Could you check a few things on this model? Use its own coordinates, in mm. A direction names the side the tool comes from. Coordinates: 2 decimals unless noted, no trailing zeros. Order: outer loops, then holes, each group sorted by start corner. A loop starts at its lowest first (then second) coordinate and runs counter-clockwise, first axis right, second up. Notation, with made-up numbers: (-33.75, 33) - (-14.75, 33) arc R23 cw to (-14.75, 56) - close; hole circle Ø6 at (-15.75, 74.5). An arc over 180 degrees is marked (long way). One line per item, written item: value.
from build123d import *

# Parameters (mm, degrees)
BODY_SKETCH_W       = 32
BODY_SKETCH_H       = 26.7
BODY_DEPTH          = 12.7
NUT_X_SKETCH_W      = 16.75
NUT_X_SKETCH_H      = 9.45
NUT_X_SKETCH_2_W    = 16.75
NUT_X_SKETCH_2_H    = 9.45
SOCKET_X_SKETCH_W   = 17.8
SOCKET_X_SKETCH_H   = 4.7625
SOCKET_X_SKETCH_2_W = 17.8
SOCKET_X_SKETCH_2_H = 4.7625


with BuildPart() as part:
    # Body Sketch → Body (new, symmetric)
    with BuildSketch(Plane.XY):
        with Locations((0, 0.65)):
            Rectangle(BODY_SKETCH_W, BODY_SKETCH_H)
    extrude(amount=BODY_DEPTH, both=True)

    # Nut _X Sketch → Nut _X (revolve)
    with BuildSketch(Plane.XY, mode=Mode.PRIVATE) as nut_x_sk:
        with Locations((24.375, 4.725)):
            Rectangle(NUT_X_SKETCH_W, NUT_X_SKETCH_H)
    revolve(nut_x_sk.sketch.rotate(Axis((-1000, 0, 0), (1, 0, 0)), 90), axis=Axis((-1000, 0, 0), (1, 0, 0)))

    # Nut -X Sketch 2 → Nut -X 2 (revolve)
    with BuildSketch(Plane.XY, mode=Mode.PRIVATE) as nut_x_2_sk:
        with Locations((-24.375, 4.725)):
            Rectangle(NUT_X_SKETCH_2_W, NUT_X_SKETCH_2_H)
    revolve(nut_x_2_sk.sketch.rotate(Axis((-1000, 0, 0), (1, 0, 0)), 90), axis=Axis((-1000, 0, 0), (1, 0, 0)))

    # Socket _X Sketch → Socket _X (revolve, cut)
    with BuildSketch(Plane.XY, mode=Mode.PRIVATE) as socket_x_sk:
        with Locations((24.85, 2.38125)):
            Rectangle(SOCKET_X_SKETCH_W, SOCKET_X_SKETCH_H)
    revolve(socket_x_sk.sketch.rotate(Axis((-1000, 0, 0), (1, 0, 0)), 90), axis=Axis((-1000, 0, 0), (1, 0, 0)), mode=Mode.SUBTRACT)

    # Socket -X Sketch 2 → Socket -X 2 (revolve, cut)
    with BuildSketch(Plane.XY, mode=Mode.PRIVATE) as socket_x_2_sk:
        with Locations((-24.85, 2.38125)):
            Rectangle(SOCKET_X_SKETCH_2_W, SOCKET_X_SKETCH_2_H)
    revolve(socket_x_2_sk.sketch.rotate(Axis((-1000, 0, 0), (1, 0, 0)), 90), axis=Axis((-1000, 0, 0), (1, 0, 0)), mode=Mode.SUBTRACT)

    # Stem Sketch → Stem (revolve)
    with BuildSketch(Plane.XY, mode=Mode.PRIVATE) as stem_sk:
        Polygon((0, 14), (8.5, 14), (8.5, 38), (3, 38), (3, 70.6), (0, 70.6), align=None)
    revolve(stem_sk.sketch.rotate(Axis((0, -500, 0), (0, 1, 0)), 90), axis=Axis((0, -500, 0), (0, 1, 0)))


solid = part.part
Item 1: If I drill on probe 1 along Y at (x, z) = (-26.25, 0); probe 2 along X at (y, z) = (1.5, 11.25); probe 3 along Y at (x, z) = (-6, -0.75), over which ranges is the centre line in solid material (lowest first)?
Conclusion:
probe 1: -9.45 to -4.76, 4.76 to 9.45
probe 2: -16 to 16
probe 3: -12.7 to 38
Item 2: I want a section at A-A on x = 0. Please give me the cut outline in (y, z), then the cut area to 3 significant figures.
Conclusion:
outline: (-12.7, -12.7) - (14, -12.7) - (14, -8.5) - (38, -8.5) - (38, -3) - (70.6, -3) - (70.6, 3) - (38, 3) - (38, 8.5) - (14, 8.5) - (14, 12.7) - (-12.7, 12.7) - close
area: 1,280 mm²
Item 3: Thinking about a two-plate mould opening in Z: for faces 5 (the face through (15.95, 0, 0)), 6 (the face through (-24.23, 4.65, -1.03)), 7 (the face through (-16, 9.4, 3)), 8 (the face through (-0.9, 54.53, -2.86)), which applies, pulls with the +Z half, pulls with the -Z half, needs draft (parallel to the pull), parting line crosses it, or undercut?
Conclusion:
face 5: undercut
face 6: undercut
face 7: needs draft
face 8: parting line crosses it
Item 4: I want a section at C-C on z = 0. Please give me the cut outline in (x, y).
Conclusion:
outline: (-32.75, -9.45) - (-16, -9.45) - (-16, -12.7) - (16, -12.7) - (16, -9.45) - (32.75, -9.45) - (32.75, -4.76) - (15.95, -4.76) - (15.95, 4.76) - (32.75, 4.76) - (32.75, 9.45) - (16, 9.45) - (16, 14) - (8.5, 14) - (8.5, 38) - (3, 38) - (3, 70.6) - (-3, 70.6) - (-3, 38) - (-8.5, 38) - (-8.5, 14) - (-16, 14) - (-16, 9.45) - (-32.75, 9.45) - (-32.75, 4.76) - (-15.95, 4.76) - (-15.95, -4.76) - (-32.75, -4.76) - close
Item 5: I'm going to push flat-ended pins straight in: pin 1 Ø6 at (x, z) = (25, -8) entering from +Y; pin 2 Ø8.5 at (y, z) = (0, 0) entering from -X. Where does each tip first touch, or does it pass through?
Conclusion:
pin 1: y = 8.02
pin 2: x = -15.95
Item 6: For faces 1 (the face through (-15.95, 0, 0)), 2 (the face through (24.492, -2.839, 9.014)), 3 (the face through (0, -12.7, 0)), 4 (the face through (-8.428, 26.168, 1.107)), which set-ups out of +Z, -Z, +X, -X, +Y, -Y let a thin tool reach every point of the face, with its end or its side?
Conclusion:
face 1: -X
face 2: +X
face 3: +Z, -Z, +X, -X, -Y
face 4: +Y
Item 7: I want a section at B-B on y = 0. Please give me the cut outline in (x, z), then the cut area to 3 significant figures.
Conclusion:
outline: (-32.75, -9.45) - (-16, -9.45) - (-16, -12.7) - (16, -12.7) - (16, -9.45) - (32.75, -9.45) - (32.75, -4.76) - (15.95, -4.76) - (15.95, 4.76) - (32.75, 4.76) - (32.75, 9.45) - (16, 9.45) - (16, 12.7) - (-16, 12.7) - (-16, 9.45) - (-32.75, 9.45) - (-32.75, 4.76) - (-15.95, 4.76) - (-15.95, -4.76) - (-32.75, -4.76) - close
area: 1,130 mm²
